Model file for the job. Use its own axes, mm. Face numbers are marked on the shaded views. A direction names the side the tool comes from. Round coordinates to 2 decimals unless told otherwise and drop trailing zeros. Write each loop counter-clockwise with the first axis right and the second up, starting at its lowest first coordinate (ties: lowest second). Pieces come first, ordered by that corner, then holes. Notation, with made-up numbers: (75, -15.75) - (86, -15.75) arc R8 cw to (86, -11.75) - close; hole circle Ø11 at (34.5, 22). An arc over 180 degrees is marked (long way). One line per item, written item: value.
Solid Edge part; units mm, degrees
sketch "Sketch1" plane through (0, 0, 0) normal (1, 0, 0) x (0, 1, 0)
  line L0 (-23.5556, 21) -> (-23.5556, 90)
  line L1 (-23.5556, 90) -> (-20.5556, 90)
  line L2 (-20.5556, 90) -> (-20.5556, 80)
  line L3 (-20.5556, 80) -> (-5.5556, 80)
  line L4 (-5.5556, 80) -> (-5.5556, 30)
  line L5 (-5.5556, 30) -> (9.4444, 30)
  line L6 (9.4444, 30) -> (9.4444, 21)
  line L7 (9.4444, 21) -> (-23.5556, 21)
  dimension "D1" = 23.5556
  dimension "D2" = 20.5556
  dimension "D3" = 5.5556
  dimension "D4" = 20.5556
  dimension "D5" = 5.5556
revolve "RevolvedProtrusion1" add sketch "Sketch1" angle 360 about axis through (0, -60, 0) along (0, 1, 0)
sketch "Sketch2" plane through (0, -5.5556, 0) normal (0, 1, 0) x (-1, 0, 0)
  line L0 (-4, 40.4732) -> (4, 40.4732)
  line L1 (4, 40.4732) -> (4, -40.4732)
  line L2 (4, -40.4732) -> (-4, -40.4732)
  line L3 (-4, -40.4732) -> (-4, 40.4732)
  dimension "D1" = 4
  dimension "D2" = 4
extrude "Cutout1" cut sketch "Sketch2" along normal blind 383.6956
hole "Hole_2" at (0, 5.0428, 0) direction (1, 0, 0) diameter 5.8 end up to next
hole "Hole_3" at (0, 5.0428, 0) direction (-1, 0, 0) diameter 5.8 end up to next
sketch "Sketch3" plane through (0, -5.5556, 0) normal (0, 1, 0) x (-1, 0, 0)
  circle A0 centre (0, -54) radius 15
  circle A1 centre (0, 54) radius 15
  circle A2 centre (38.2737, -38) radius 15
  circle A3 centre (38.2737, 37.8947) radius 15
  circle A4 centre (-37, 37.8947) radius 15
  circle A5 centre (-37, -38) radius 15
  circle A6 centre (-55, 0) radius 15
  circle A7 centre (55, 0) radius 15
extrude "ExtrudedCutout_6" cut sketch "Sketch3" against normal blind 135.9253
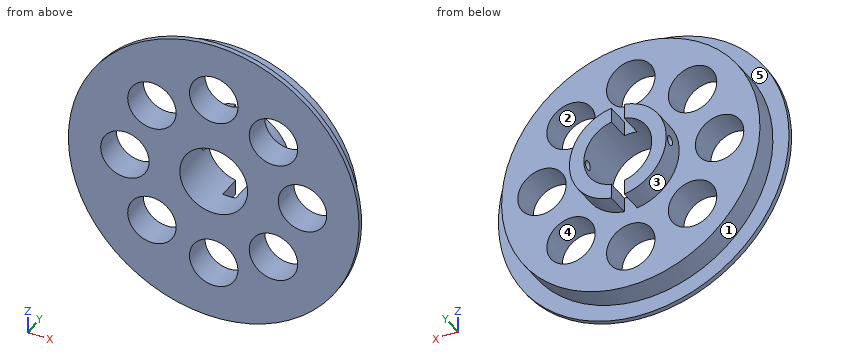
1. Mould opens along X. For the marked faces 1, 2 and 3 say: released by +X, released by -X, zero draft, split by the parting line, or undercut.
Report:
face 1: split by the parting line
face 2: undercut
face 3: released by -X
2. Band-saw the part on D-D on x = 37. Write the cut outline in (y, z).
Report:
outline: (-23.56, -82.04) - (-20.56, -82.04) - (-20.56, -70.93) - (-5.56, -70.93) - (-5.56, -53) - (-23.56, -53) - close; (-23.56, -23) - (-5.56, -23) - (-5.56, 22.89) - (-23.56, 22.89) - close; (-23.56, 52.89) - (-5.56, 52.89) - (-5.56, 70.93) - (-20.56, 70.93) - (-20.56, 82.04) - (-23.56, 82.04) - close
3. Wall check: probe 1 along Z at (x, y) = (-8, -12); probe 2 along Z at (x, y) = (37, -12.5); probe 3 along Y at (x, z) = (-26.25, 0). Give the ranges that are in metal, low to high. Write a range as [from, to].
Report:
probe 1: [-79.6, -66.69], [-41.31, -19.42], [19.42, 41.31], [66.69, 79.6]
probe 2: [-70.93, -53], [-23, 22.89], [52.89, 70.93]
probe 3: [-23.56, 2.14], [7.94, 9.44]
4. Band-saw the part on C-C on z = 63.5. Write the cut outline in (x, y), plus the area to 3 significant figures.
Report:
outline: (-63.78, -23.56) - (-11.61, -23.56) - (-11.61, -5.56) - (-48.66, -5.56) - (-48.66, -20.56) - (-63.78, -20.56) - close; (11.61, -23.56) - (63.78, -23.56) - (63.78, -20.56) - (48.66, -20.56) - (48.66, -5.56) - (11.61, -5.56) - close
area: 1,420 mm²
5. Tool access for the marked faces 4 and 5: list every direction of +Z, -Z, +X, -X, +Y, -Y with a clear straight run to the whole face (end or side of a thin tool).
Report:
face 4: +Y, -Y
face 5: +Y
6. Band-saw the part on B-B on z = 0. State how many separate pieces and enclosed holes the cut face has, plus the area to 3 significant figures.
Report:
separate pieces: 6
enclosed holes: 0
area: 1,270 mm²
7. Band-saw the part on A-A on x = 0. Write the cut outline in (y, z), plus the area to 3 significant figures.
Report:
outline: (-23.56, -90) - (-20.56, -90) - (-20.56, -80) - (-5.56, -80) - (-5.56, -69) - (-23.56, -69) - close; (-23.56, -39) - (-5.56, -39) - (-5.56, -21) - (-23.56, -21) - close; (-23.56, 21) - (-5.56, 21) - (-5.56, 39) - (-23.56, 39) - close; (-23.56, 69) - (-5.56, 69) - (-5.56, 80) - (-20.56, 80) - (-20.56, 90) - (-23.56, 90) - close
area: 1,100 mm²
8. Drop flat-ended pins along their axis: pin 1 (1 mm diameter, centred on x = 26.5, y = -2, fed in from +Z); pin 2 (10 mm diameter, centred on x = 11, y = -17, fed in from +Z); pin 3 (6 mm diameter, centred on x = -38.5, z = 28, fed in from -Y); pin 4 (10 mm diameter, centred on y = 0, z = 26.5, fed in from +X). Give the stop position or say it passes through.
Report:
pin 1: z = 14.97
pin 2: z = 89.69
pin 3: through
pin 4: x = 20.92
